```python
from build123d import *

# Parameters (mm, degrees)
F3_DEPTH        = 73.66
F3_COPIES_COUNT = 3
F4_R            = 0.4


# Not quite as in the source:
# - a pattern or mirror of a feature is missing from the dataset's text; its kind, count and spacing are read off the source's solid


with BuildPart() as f1:
    # F0 (on Front) → F1 (revolve)
    with BuildSketch(Plane.XZ):
        Polygon((28.7253968418, 54.2925000191), (0, 54.2925000191), (0, 47.6751327515), (16.0922370851, 47.6751327515), (16.0922370851, 42.5617098808), (28.7253968418, 42.5617098808), align=None)
    revolve(axis=Axis((14.3626984209, 0, 0), (1, 0, 0)))

    # F2 (on Top) → F3 (cut)
    with BuildSketch(Plane.XY):
        with BuildLine():
            Line((1.6697708597, 4.963026382), (0, 4.963026382))
            Line((0, 4.963026382), (-7.0685544051, 4.963026382))
            Line((-7.0685544051, 4.963026382), (-7.0685544051, -4.963026382))
            Line((-7.0685544051, -4.963026382), (0, -4.963026382))
            Line((0, -4.963026382), (1.6697708597, -4.963026382))
            ThreePointArc((1.6697708597, -4.963026382), (5.8676445687, 0), (1.6697708597, 4.963026382))
        make_face()
    f3 = extrude(amount=F3_DEPTH, mode=Mode.SUBTRACT)

    # F3_copies: F3 ×3 about axis
    f3_copies_axis = Axis((0, 0, 0), (1, 0, 0))
    for i in range(1, F3_COPIES_COUNT):
        add(f3.rotate(f3_copies_axis, i * 360 / F3_COPIES_COUNT), mode=Mode.SUBTRACT)

    # F4
    f4_edges = [f1.edges().sort_by_distance(p)[0] for p in [
        (16.092237, 0, -47.675133),
    ]]
    fillet(f4_edges, radius=F4_R)


solid = f1.part
```
The model under review builds one solid part; all positions refer to its coordinate system, in mm. A direction names the side the tool comes from. Give positions to 0.01 mm unless a question says otherwise; leave off trailing zeros. Order: outer loops, then holes, each group sorted by start corner. A loop starts at its lowest first (then second) coordinate and runs counter-clockwise, first axis right, second up. Notation, with made-up numbers: (83.5, -12) - (127.5, -12) arc R10 ccw to (127.5, -5) - close; hole circle Ø3 at (46, -38.75). An arc over 180 degrees is marked (long way). Use CSV: the item, a comma, the result in double quotes. Start each with the question number.
Q1. We need section A-A, the plane z = 0. Write out the cut boundary in (x, y), and give its area (3 significant figures).
Q2. To check wall thickness, follow line 1 along Y through (x, z) = (20, 0); line 2 along Y through (x, z) = (8, 0). State the ranges of each line that lie inside material, in increasing order. Write a range as [from, to].
Q3. We need section C-C, the plane x = 10.25. Write out the cut boundary in (y, z) (1 decimal).
Q4. Tool access review of faces 5 (the flat face through (0.847, 41.421, -29.645)), 6 (the flat face through (16.092, -18, -39)), 7 (the flat face through (0.823, -41.421, -29.645)): name each direction out of +Z, -Z, +X, -X, +Y, -Y from which nothing blocks a thin tool from reaching the whole face with its end or side.
Q5. The part is to be moulded in two halves that separate along Z. For faces 1 (the cylindrical face through (5.867, -43.953, -25.49)), 2 (the cylindrical face through (22.497, 25.898, -33.776)), 3 (the cylindrical face through (14.16, 33.04, -43.08)), 4 (the flat face through (0, 42, 24)), say which applies: +Z half, -Z half, draft (parallel to the pull), parting line (faces both ways), or undercut.
Q6. We need section D-D, the plane x = 17.5. Write out the cut boundary in (y, z) (1 decimal).
Q7. Clearance check with flat-ended pins moving along their axes: pin 1 Ø1.3 at (x, z) = (1, 50) entering from -Y; pin 2 Ø10 at (x, z) = (14, 8) entering from -Y; pin 3 Ø8 at (x, z) = (25, -20.5) entering from +Y; pin 4 Ø3 at (y, z) = (-37.5, -19) entering from +X. State where each tip first meets the part, or that it passes through.
Q8. We need section B-B, the plane y = 0. Write out the cut boundary in (x, z).
Outcome:
1,outline,"(0, -54.29) - (28.73, -54.29) - (28.73, -42.56) - (16.09, -42.56) - (16.09, -47.28) arc R0.4 cw to (15.69, -47.68) - (0, -47.68) - close; (0, 47.68) - (15.69, 47.68) arc R0.4 cw to (16.09, 47.28) - (16.09, 42.56) - (28.73, 42.56) - (28.73, 54.29) - (0, 54.29) - close"
1,area,"509 mm^2"
2,line 1,"y = [-54.29, -42.56], [42.56, 54.29]"
2,line 2,"y = [-54.29, -47.68], [47.68, 54.29]"
3,outline,"circle Ø108.6 at (0, 0); hole circle Ø95.4 at (0, 0)"
4,face 5,"-X, +Y"
4,face 6,"-X"
4,face 7,"-X, -Y"
5,face 1,"undercut"
5,face 2,"undercut"
5,face 3,"parting line"
5,face 4,"draft"
6,outline,"circle Ø108.6 at (0, 0); hole circle Ø85.1 at (0, 0)"
7,pin 1,"stops at y = -22.63"
7,pin 2,"stops at y = -54.21"
7,pin 3,"stops at y = 51.72"
7,pin 4,"stops at x = 28.73"
8,outline,"(0, -54.29) - (28.73, -54.29) - (28.73, -42.56) - (16.09, -42.56) - (16.09, -47.28) arc R0.4 cw to (15.69, -47.68) - (0, -47.68) - close; (5.87, 47.68) - (15.69, 47.68) arc R0.4 cw to (16.09, 47.28) - (16.09, 42.56) - (28.73, 42.56) - (28.73, 54.29) - (5.87, 54.29) - close"
